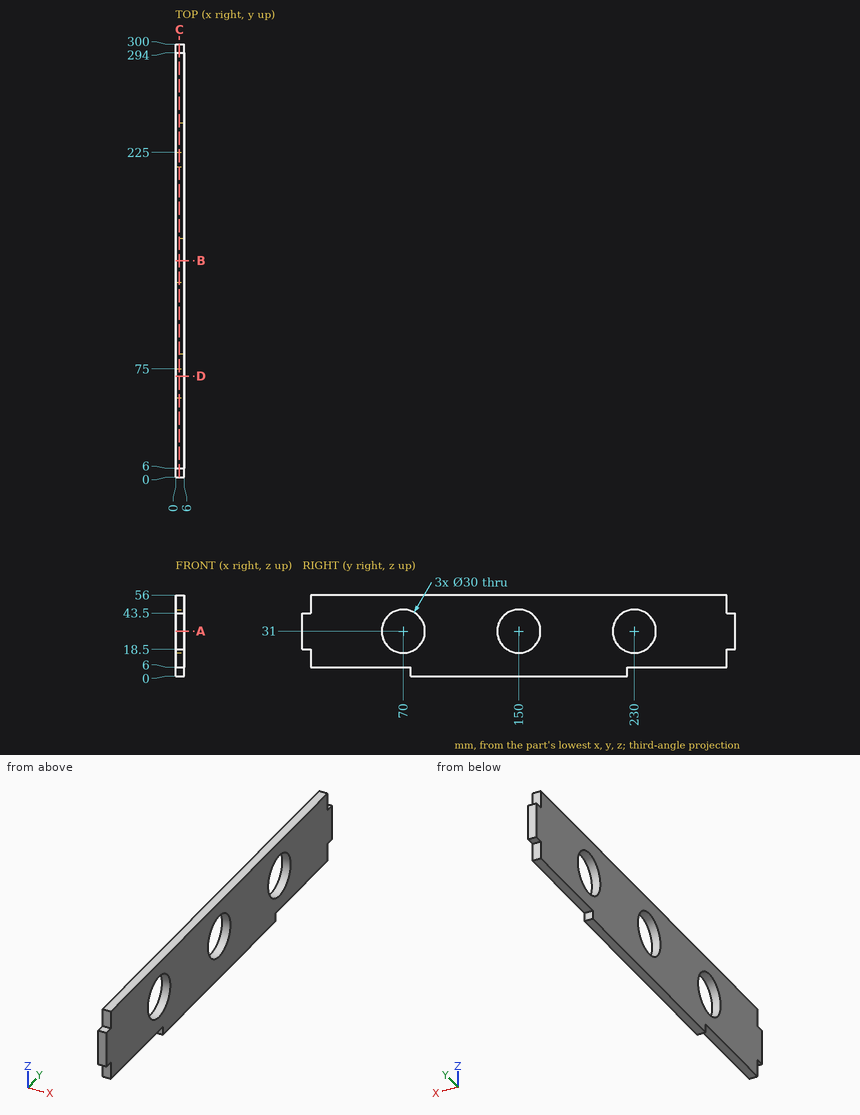
Study the drawing (mm; zero at the part's minimum x, y, z) and answer. Round coordinates to 2 decimals unless told otherwise and drop trailing zeros. Order: outer loops, then holes, each group sorted by start corner. A loop starts at its lowest first (then second) coordinate and runs counter-clockwise, first axis right, second up. Notation, with made-up numbers: (80, -13.5) - (93, -13.5) arc R35 cw to (93, 18.5) - close; hole circle Ø1 at (-2, 22). An arc over 180 degrees is marked (long way). Use one line per item in the form item = value. Start each with the question number.
(1) The part is cut by section C-C (x = 2.65). Give the vertices of the cut face in (y, z).
(2) The part is cut by section A-A (z = 31). Give the vertices of the cut face in (x, y).
(3) Flat-ended cylindrical pins translate along their axes: pin 1 Ø1.8 at (x, z) = (3, 9.5) entering from +Y; pin 2 Ø3 at (x, z) = (2, 2.5) entering from +Y; pin 3 Ø3 at (x, y) = (3.5, 199.5) entering from -Z; pin 4 Ø1.8 at (x, y) = (2.5, 43) entering from -Z. Find the tip coordinate at first contact, or state that the pin passes through.
(4) Find the intervals of material crossed by line 1 along Z through (x, y) = (2, 150); line 2 along Y through (x, z) = (5.05, 35); line 3 along Y through (x, z) = (3.95, 37.5), in increasing order. Write a range as from..to.
(5) The part is cut by section B-B (y = 150). Give the vertices of the cut face in (x, z).
(6) The part is cut by section D-D (y = 70). Give the vertices of the cut face in (x, z).
Checked values:
q1.outline = (0, 18.5) - (6, 18.5) - (6, 6) - (75, 6) - (75, 0) - (225, 0) - (225, 6) - (294, 6) - (294, 18.5) - (300, 18.5) - (300, 43.5) - (294, 43.5) - (294, 56) - (6, 56) - (6, 43.5) - (0, 43.5) - close; hole circle Ø30 at (70, 31); hole circle Ø30 at (150, 31); hole circle Ø30 at (230, 31)
q2.outline = (0, 0) - (6, 0) - (6, 55) - (0, 55) - close; (0, 85) - (6, 85) - (6, 135) - (0, 135) - close; (0, 165) - (6, 165) - (6, 215) - (0, 215) - close; (0, 245) - (6, 245) - (6, 300) - (0, 300) - close
q3.pin_1 = 294
q3.pin_2 = 225
q3.pin_3 = 0
q3.pin_4 = 6
q4.line_1 = 0..16, 46..56
q4.line_2 = 0..55.54, 84.46..135.54, 164.46..215.54, 244.46..300
q4.line_3 = 0..56.48, 83.52..136.48, 163.52..216.48, 243.52..300
q5.outline = (0, 0) - (6, 0) - (6, 16) - (0, 16) - close; (0, 46) - (6, 46) - (6, 56) - (0, 56) - close
q6.outline = (0, 6) - (6, 6) - (6, 16) - (0, 16) - close; (0, 46) - (6, 46) - (6, 56) - (0, 56) - close
